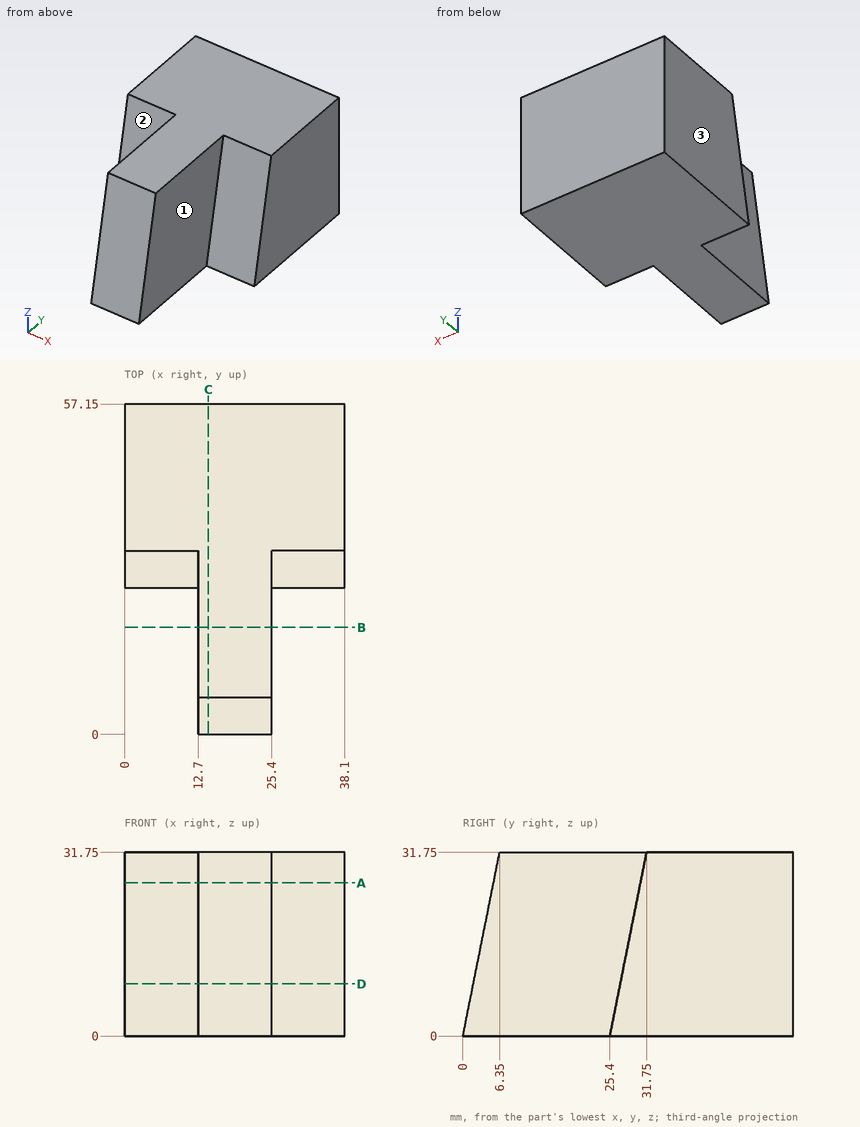
Part print with two shaded views. Sizes in mm from the minimum x, y, z corner. A direction names the side the tool comes from. Round coordinates to 2 decimals unless told otherwise and drop trailing zeros. Write each loop counter-clockwise with the first axis right and the second up, starting at its lowest first coordinate (ties: lowest second). Pieces come first, ordered by that corner, then holes. Notation, with made-up numbers: (66, 52) - (114, 52) arc R8 cw to (114, 60) - close; hole circle Ø1 at (-7.75, 59). An arc over 180 degrees is marked (long way). Answer as CSV lines item,"result".
Q1. Drop flat-ended pins along their axis: pin 1 (16 mm diameter, centred on y = 12, z = 20.5, fed in from +X); pin 2 (6 mm diameter, centred on y = 41, z = 6.5, fed in from -X); pin 3 (16 mm diameter, centred on y = 18, z = 9.5, fed in from -X); pin 4 (2 mm diameter, centred on x = 27, z = 27.5, fed in from -Y). Give the stop position or say it passes through.
Report:
pin 1,"stops at x = 25.4"
pin 2,"stops at x = 0"
pin 3,"stops at x = 12.7"
pin 4,"stops at y = 30.7"
Q2. Cut at C-C (x = 14.5). Write the cut outline in (y, z), and give its area (3 significant figures).
Report:
outline,"(0, 0) - (57.15, 0) - (57.15, 31.75) - (6.35, 31.75) - close"
area,"1,710 mm^2"
Q3. Cut at B-B (y = 18.5). Write the cut outline in (x, z), and give its area (3 significant figures).
Report:
outline,"(12.7, 0) - (25.4, 0) - (25.4, 31.75) - (12.7, 31.75) - close"
area,"403 mm^2"
Q4. Cut at D-D (z = 9). Write the cut outline in (x, y), and give its area (3 significant figures).
Report:
outline,"(0, 27.2) - (12.7, 27.2) - (12.7, 1.8) - (25.4, 1.8) - (25.4, 27.2) - (38.1, 27.2) - (38.1, 57.15) - (0, 57.15) - close"
area,"1,460 mm^2"
Q5. Drill centre lines: probe 1 along X at (y, z) = (18.5, 2.5); probe 2 along Y at (x, z) = (32.5, 23); probe 3 along Y at (x, z) = (2.5, 18.5). Where is each one in solid material? Low to high. Write a range as [from, to].
Report:
probe 1,"x = [12.7, 25.4]"
probe 2,"y = [30, 57.15]"
probe 3,"y = [29.1, 57.15]"
Q6. Tool access for the marked faces 1, 2 and 3: list every direction of +Z, -Z, +X, -X, +Y, -Y with a clear straight run to the whole face (end or side of a thin tool).
Report:
face 1,"+Z, +X, -Y"
face 2,"+Z, -X, -Y"
face 3,"+Z, -Z, -X, +Y, -Y"
Q7. Cut at A-A (z = 26.5). Write the cut outline in (x, y).
Report:
outline,"(0, 30.7) - (12.7, 30.7) - (12.7, 5.3) - (25.4, 5.3) - (25.4, 30.7) - (38.1, 30.7) - (38.1, 57.15) - (0, 57.15) - close"
